Geometry check sheet. Reference: drawing and pictorial views, mm from the part's lowest x, y, z. Round coordinates to 2 decimals unless told otherwise and drop trailing zeros. Order: outer loops, then holes, each group sorted by start corner. A loop starts at its lowest first (then second) coordinate and runs counter-clockwise, first axis right, second up.
(1) Sectioned sample at A-A (x = 83). Record the boundary of the cut face in (y, z).
(2) Sectioned sample at D-D (x = 15). Record the boundary of the cut face in (y, z), plus the area to 3 significant figures.
(3) Sectioned sample at C-C (z = 10.5). Record the boundary of the cut face in (x, y).
(4) Release check for a two-part mould opening along X. For the marked faces 1 and 2 record: +X half, -X half, draft (parallel to the pull), parting line (faces both ways), or undercut.
(5) Material ranges on line 1 along X through (y, z) = (33.5, 33); line 2 along X through (y, z) = (108, 5); line 3 along Y through (x, z) = (75.5, 16), recorded low to high.
(6) Go/stop test with flat-tipped pins: pin 1 (4 mm diameter, centred on y = 85.5, z = 29.5, fed in from +X); pin 2 (19 mm diameter, centred on y = 90, z = 21, fed in from -X); pin 3 (6 mm diameter, centred on x = 79.5, z = 29.5, fed in from -Y); pin 4 (4 mm diameter, centred on y = 119, z = 9, fed in from +X). Record where each tip stops, or that it passes through.
(7) Sectioned sample at B-B (y = 88.5). Record the boundary of the cut face in (x, z).
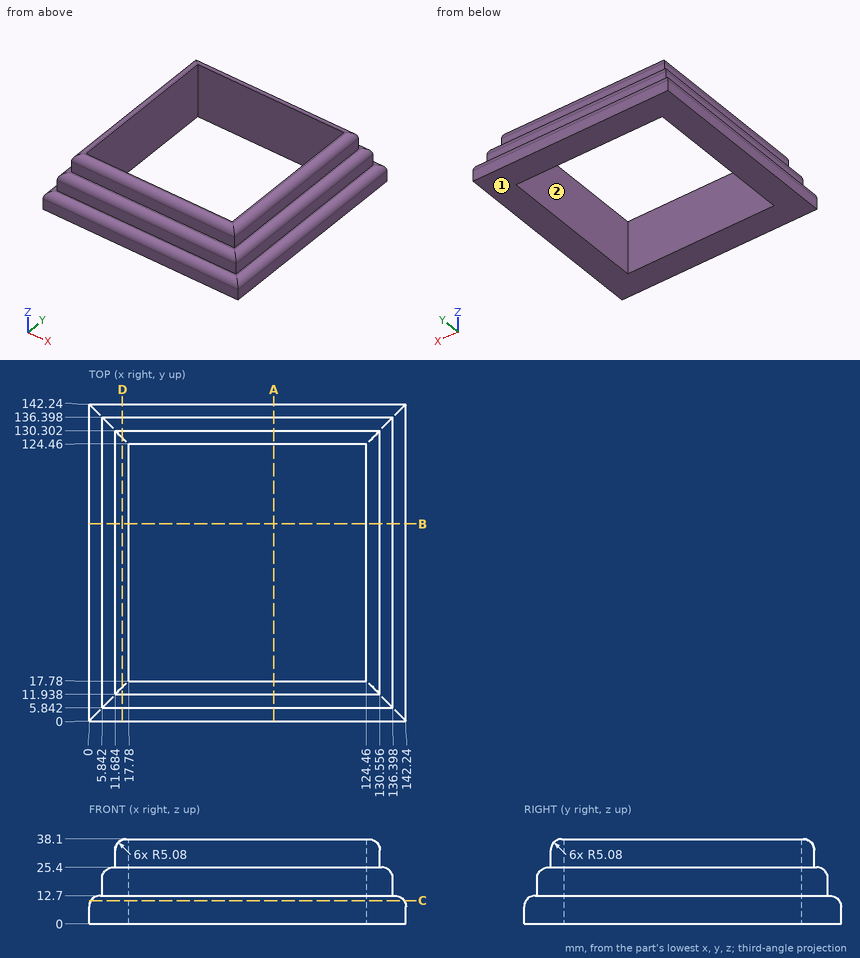
Answer below:
1. outline: (0, 0) - (17.78, 0) - (17.78, 38.1) - (17.02, 38.1) arc R5.08 ccw to (11.94, 33.02) - (11.94, 25.4) - (10.92, 25.4) arc R5.08 ccw to (5.84, 20.32) - (5.84, 12.7) - (5.08, 12.7) arc R5.08 ccw to (0, 7.62) - close; (124.46, 0) - (142.24, 0) - (142.24, 7.62) arc R5.08 ccw to (137.16, 12.7) - (136.4, 12.7) - (136.4, 20.32) arc R5.08 ccw to (131.32, 25.4) - (130.3, 25.4) - (130.3, 33.02) arc R5.08 ccw to (125.22, 38.1) - (124.46, 38.1) - close
2. outline: (0, 0) - (142.24, 0) - (142.24, 7.62) arc R5.08 ccw to (137.16, 12.7) - (136.4, 12.7) - (136.4, 20.32) arc R5.08 ccw to (131.32, 25.4) - (130.3, 25.4) - (130.3, 33.02) arc R5.08 ccw to (126.99, 37.78) - (15.25, 37.78) arc R5.08 ccw to (11.94, 33.02) - (11.94, 25.4) - (10.92, 25.4) arc R5.08 ccw to (5.84, 20.32) - (5.84, 12.7) - (5.08, 12.7) arc R5.08 ccw to (0, 7.62) - close
2. area: 4,900 mm2
3. outline: (0.9, 0.9) - (141.34, 0.9) - (141.34, 141.34) - (0.9, 141.34) - close; hole (17.78, 17.78) - (124.46, 17.78) - (124.46, 124.46) - (17.78, 124.46) - close
4. face 1: draft
4. face 2: undercut
5. line 1: x = 11.68 to 17.78, 124.46 to 130.56
5. line 2: x = 0 to 17.78, 124.46 to 142.24
5. line 3: y = 5.84 to 17.78, 124.46 to 136.4
6. pin 1: stops at x = 130.56
6. pin 2: stops at x = 1.8
6. pin 3: stops at y = 11.94
6. pin 4: stops at x = 142.24
7. outline: (0, 0) - (17.78, 0) - (17.78, 38.1) - (16.76, 38.1) arc R5.08 ccw to (11.68, 33.02) - (11.68, 25.4) - (10.92, 25.4) arc R5.08 ccw to (5.84, 20.32) - (5.84, 12.7) - (5.08, 12.7) arc R5.08 ccw to (0, 7.62) - close; (124.46, 0) - (142.24, 0) - (142.24, 7.62) arc R5.08 ccw to (137.16, 12.7) - (136.4, 12.7) - (136.4, 20.32) arc R5.08 ccw to (131.32, 25.4) - (130.56, 25.4) - (130.56, 33.02) arc R5.08 ccw to (125.48, 38.1) - (124.46, 38.1) - close
